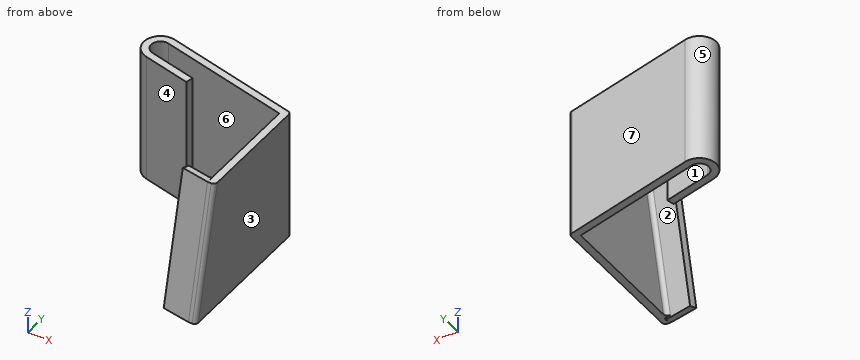
from build123d import *

# Parameters (mm, degrees)
EXTRUS_O_FINA1_DEPTH     = 35
RESSALTO_EXTRUS_O1_DEPTH = 2
ESBO_O4_W                = 35.902646142
ESBO_O4_H                = 2
EXTRUS_O_FINA2_DEPTH     = 8
FILETE1_R                = 1


with BuildPart() as part:
    # Esboço1 → Extrusão-Fina1 (new body)
    with BuildSketch(Plane.XY):
        with BuildLine():
            Line((0, -9.06918845), (0, 20.93081155))
            Line((0, 20.93081155), (-35.077322332, 29.029049507))
            ThreePointArc((-35.077322332, 29.029049507), (-38.07562513, 27.155501981), (-36.202077604, 24.157199183))
            Line((-36.202077604, 24.157199183), (-23.535266762, 21.232835476))
            Line((-23.535266762, 21.232835476), (-23.98516887, 19.284095347))
            Line((-23.98516887, 19.284095347), (-36.651979713, 22.208459053))
            ThreePointArc((-36.651979713, 22.208459053), (-40.02436526, 27.605404089), (-34.627420224, 30.977789636))
            Line((-34.627420224, 30.977789636), (2, 22.521683384))
            Line((2, 22.521683384), (2, -9.06918845))
            Line((2, -9.06918845), (0, -9.06918845))
        make_face()
    extrude(amount=EXTRUS_O_FINA1_DEPTH)

    # Esboço2 → Ressalto-extrusão1 (add)
    with BuildSketch(Plane(origin=(0, 0, 0), x_dir=(0, 0, -1), z_dir=(1, 0, 0))):
        Polygon((0, -9.06918845), (-35, -9.06918845), (0, -17.06918845), align=None)
    extrude(amount=RESSALTO_EXTRUS_O1_DEPTH)

    # Esboço4 → Extrusão-Fina2 (add)
    with BuildSketch(Plane(origin=(3.647257489, -0.820865703, 0.187626446), x_dir=(0, 0.2228248015021411, 0.9748585065718673), z_dir=(0.9743700647852352, -0.21929544888942776, 0.050124674031869196))):
        with Locations((14.147884543, 15.213560322)):
            Rectangle(ESBO_O4_W, ESBO_O4_H)
    extrude(amount=-EXTRUS_O_FINA2_DEPTH)

    # Filete1
    filete1_edges = [part.edges().sort_by_distance(p)[0] for p in [
        (2, 22.521683384, 17.5),
        (2, -13.06918845, 17.5),
        (0, -11.015914782, 17.271313991),
    ]]
    fillet(filete1_edges, radius=FILETE1_R)


solid = part.part
Input: part model. Units: mm. Frame: model coordinates. Face numbers are marked on the shaded views. A direction names the side the tool comes from. Coordinates: 2 decimals unless noted, no trailing zeros. Loops run counter-clockwise (first coordinate to the right, second up) from the corner with the lowest first, then second, coordinate; pieces in that order, holes last. Notation, with made-up numbers: (-37, -24) -> (-9, -24) arc R27 cw to (-9, -8) -> close; hole circle Ø5 at (35.25, 81.5). An arc over 180 degrees is marked (long way). One line per item, written item: value.
(1) Cut plane D-D (x = -22). Output: boundary loops of the cut face in (y, z), then the cut area to 3 significant figures.
Answer below:
outline: (26.01, 0) -> (28.06, 0) -> (28.06, 35) -> (26.01, 35) -> close
area: 71.8 mm2
(2) Cut plane B-B (x = -6). Output: boundary loops of the cut face in (y, z).
Answer below:
outline: (-15.72, -0.31) -> (-13.72, -0.77) -> (-5.72, 34.23) -> (-7.72, 34.69) -> close; (22.32, 0) -> (24.37, 0) -> (24.37, 35) -> (22.32, 35) -> close
(3) Cut plane C-C (y = -1.5). Output: boundary loops of the cut face in (x, z), then the cut area to 3 significant figures.
Answer below:
outline: (0, 0) -> (2, 0) -> (2, 35) -> (0, 35) -> close
area: 70.0 mm2
(4) Pin query (flat end, axial travel): pin 1 Ø2 at (x, z) = (-31, 4) entering from -Y; pin 2 Ø1.5 at (x, z) = (-20.5, 10.5) entering from +Y; pin 3 Ø1.5 at (x, z) = (-7, 23) entering from +Y. Return the tip coordinate at first contact, or that it passes through.
Answer below:
pin 1: stops at y = 20.67
pin 2: stops at y = 27.89
pin 3: stops at y = 24.77
(5) Cut plane A-A (y = 25). Output: boundary loops of the cut face in (x, z).
Answer below:
outline: (-39.85, 0) -> (-37.57, 0) -> (-37.57, 35) -> (-39.85, 35) -> close; (-17.63, 0) -> (-8.73, 0) -> (-8.73, 35) -> (-17.63, 35) -> close
(6) Draft query along Y for the marked faces 4, 5, 6 and 7. Return one class per face: pulls with the +Y half, pulls with the -Y half, needs draft (parallel to the pull), parting line crosses it, or undercut.
Answer below:
face 4: pulls with the -Y half
face 5: parting line crosses it
face 6: undercut
face 7: pulls with the +Y half
(7) Set-up query: the marked faces 1, 2 and 3. Return all of +Z, -Z, +X, -X, +Y, -Y with unobstructed straight access to the full face (end or side cutting, diameter ignored); none if empty.
Answer below:
face 1: +Z, -Z
face 2: -Z
face 3: +Z, -Z, +X, +Y, -Y
(8) Ray query, line 1 along X through (y, z) = (3.5, 28); line 2 along Y through (x, z) = (-28, 32.5); line 3 along Y through (x, z) = (-25, 30.5). Return the intervals inside material, ascending.
Answer below:
line 1: x = 0 to 2
line 2: y = 20.21 to 22.26, 27.4 to 29.45
line 3: y = 19.52 to 21.57, 26.7 to 28.76
